Geometry check sheet. Reference: the model listing, model coordinates, mm. A direction names the side the tool comes from. Give positions to 0.01 mm unless a question says otherwise; leave off trailing zeros. Write each loop counter-clockwise with the first axis right and the second up, starting at its lowest first coordinate (ties: lowest second). Pieces come first, ordered by that corner, then holes. Notation, with made-up numbers: (16.5, -23) -> (74.5, -23) arc R16 cw to (74.5, -5) -> close; hole circle Ø11 at (-7, 56.5). An arc over 180 degrees is marked (long way). One line per item, written item: value.
from build123d import *

# Parameters (mm, degrees)
SKETCH1_W           = 19.05
SKETCH1_H           = 38.1
SKETCH1_W_2         = 12.7
SKETCH1_H_2         = 31.75
EXTRUDE_THIN1_DEPTH = 50.8
SKETCH3_R           = 6.35
CUT_EXTRUDE2_DEPTH  = 67.295946332


with BuildPart() as part:
    # Sketch1 → Extrude-Thin1 (new body)
    with BuildSketch(Plane.XY):
        with Locations((9.525, 19.05)):
            Rectangle(SKETCH1_W, SKETCH1_H)
        with Locations((9.525, 19.05)):
            Rectangle(SKETCH1_W_2, SKETCH1_H_2, mode=Mode.SUBTRACT)
    extrude(amount=EXTRUDE_THIN1_DEPTH)

    # Sketch3 → Cut-Extrude2 (cut, through all)
    with BuildSketch(Plane.ZY):
        with Locations((25.4, 19.05)):
            Circle(SKETCH3_R)
    extrude(amount=-CUT_EXTRUDE2_DEPTH, mode=Mode.SUBTRACT)


solid = part.part
1) Scan lines: probe 1 along X at (y, z) = (19.5, 4) (3 decimals); probe 2 along Y at (x, z) = (12.75, 13) (3 decimals); probe 3 along Y at (x, z) = (1.85, 25.4). Record each from-to range of solid material in increasing order.
Verdict:
probe 1: 0 to 3.175, 15.875 to 19.05
probe 2: 0 to 3.175, 34.925 to 38.1
probe 3: 0 to 12.7, 25.4 to 38.1
2) Tool access check on faces 4 (the flat face through (3, 19, 50.8)), 5 (the flat face through (15.875, 15, 19)). Record the directions out of +Z, -Z, +X, -X, +Y, -Y that give a thin tool (end or side, any length) a straight path to the whole face; none if there is none.
Verdict:
face 4: +Z, +X, -X, +Y, -Y
face 5: +Z, -Z
3) Sectioned sample at C-C on y = 19.05. Record the cut outline in (x, z) (3 decimals), plus the area to 3 significant figures.
Verdict:
outline: (0, 0) -> (3.175, 0) -> (3.175, 19.05) -> (0, 19.05) -> close; (0, 31.75) -> (3.175, 31.75) -> (3.175, 50.8) -> (0, 50.8) -> close; (15.875, 0) -> (19.05, 0) -> (19.05, 19.05) -> (15.875, 19.05) -> close; (15.875, 31.75) -> (19.05, 31.75) -> (19.05, 50.8) -> (15.875, 50.8) -> close
area: 242 mm^2
4) Sectioned sample at B-B on x = 9.5. Record the cut outline in (y, z) (3 decimals).
Verdict:
outline: (0, 0) -> (3.175, 0) -> (3.175, 50.8) -> (0, 50.8) -> close; (34.925, 0) -> (38.1, 0) -> (38.1, 50.8) -> (34.925, 50.8) -> close
5) Mould release check, pull along X, two halves, no side actions. Record for faces 1 (the flat face through (9, 34.925, 25)), 2 (the flat face through (19.05, 23, 31)), 3 (the cylindrical face through (1.57, 23.34, 20.72)): released by +X, released by -X, zero draft, split by the parting line, or undercut.
Verdict:
face 1: undercut
face 2: released by +X
face 3: zero draft
6) Sectioned sample at D-D on z = 44. Record the cut outline in (x, y) (3 decimals), plus the area to 3 significant figures.
Verdict:
outline: (0, 0) -> (19.05, 0) -> (19.05, 38.1) -> (0, 38.1) -> close; hole (3.175, 3.175) -> (15.875, 3.175) -> (15.875, 34.925) -> (3.175, 34.925) -> close
area: 323 mm^2
7) Sectioned sample at A-A on y = 26.5. Record the cut outline in (x, z) (3 decimals), plus the area to 3 significant figures.
Verdict:
outline: (0, 0) -> (3.175, 0) -> (3.175, 50.8) -> (0, 50.8) -> close; (15.875, 0) -> (19.05, 0) -> (19.05, 50.8) -> (15.875, 50.8) -> close
area: 323 mm^2
